from build123d import *

# Parameters (mm, degrees)
F0_W     = 63.6
F0_H     = 31.8
F1_DEPTH = 9.6
F2_W     = 61.2
F2_H     = 29.4
F3_DEPTH = 8.4
F4_R     = 2
F6_DEPTH = 32


with BuildPart() as f1:
    # F0 (on Top) → F1 (new body)
    with BuildSketch(Plane.XY):
        Rectangle(F0_W, F0_H)
    extrude(amount=F1_DEPTH)

    # F2 (on Top) → F3 (cut)
    with BuildSketch(Plane.XY):
        Rectangle(F2_W, F2_H)
    extrude(amount=F3_DEPTH, mode=Mode.SUBTRACT)

    # F4
    f4_edges = [f1.edges().sort_by_distance(p)[0] for p in [
        (-31.8, -15.9, 4.8),
        (-31.8, 15.9, 4.8),
        (31.8, 15.9, 4.8),
        (31.8, -15.9, 4.8),
    ]]
    fillet(f4_edges, radius=F4_R)

    # F5 (on Right) → F6 (cut)
    with BuildSketch(Plane.YZ):
        with BuildLine():
            Line((3.71, 1.5), (-3.71, 1.5))
            ThreePointArc((-3.71, 1.5), (-4.346396, 1.236396), (-4.61, 0.6))
            Line((-4.61, 0.6), (-4.61, -0.6))
            ThreePointArc((-4.61, -0.6), (-4.346396, -1.236396), (-3.71, -1.5))
            Line((-3.71, -1.5), (3.71, -1.5))
            ThreePointArc((3.71, -1.5), (4.346396, -1.236396), (4.61, -0.6))
            Line((4.61, -0.6), (4.61, 0.6))
            ThreePointArc((4.61, 0.6), (4.346396, 1.236396), (3.71, 1.5))
        make_face()
    extrude(amount=F6_DEPTH, mode=Mode.SUBTRACT)


solid = f1.part
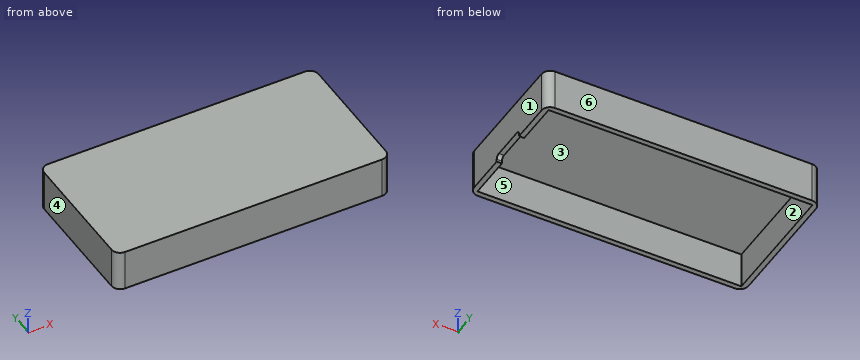
The model under review builds one solid part; all positions refer to its coordinate system, in mm. Face numbers are marked on the shaded views. A direction names the side the tool comes from. Give positions to 0.01 mm unless a question says otherwise; leave off trailing zeros. Order: outer loops, then holes, each group sorted by start corner. A loop starts at its lowest first (then second) coordinate and runs counter-clockwise, first axis right, second up. Notation, with made-up numbers: M 4.5,84 L 23.5,84 A21 ccw 23.5,88 Z; hole C -5.75,13.25 d4. An arc over 180 degrees is marked long. Answer in a Markdown table with one row per item. Add a question column.
1. Machinability: for the marked faces 1 and 2, which of the approach directions +Z, -Z, +X, -X, +Y, -Y give a long, thin tool a straight path to every point of the face, cutting with its end or side? Answer none if there is none.
2. For pin 1 Ø1 at (x, y) = (31, 1) entering from -Z; pin 2 Ø0.7 at (x, z) = (31, 0) entering from -Y; pin 3 Ø8 at (x, y) = (-9, 9.5) entering from -Z, all flat-tipped, find the tip position at first contact; note any pin that passes through.
3. Add section A-A on x = 8. State the section outline as (y, z) points, plus the area to 3 significant figures.
4. Mouldability with a two-part tool opening along X and no side actions: class the marked faces 3, 4, 5 and 6 as released by +X, released by -X, zero draft, split by the parting line, or undercut.
5. To check wall thickness, follow line 1 along X through (y, z) = (12.5, 2.5); line 2 along Y through (x, z) = (2, 4.5); line 3 along Z through (x, y) = (4, 11.5). State the ranges of each line that lie inside material, in increasing order.
6. Add section B-B on y = 8. State the section outline as (x, z) points, plus the area to 3 significant figures.
The answers:
| question | item | result |
|---|---|---|
| 1 | face 1 | +Z, -Z, +X, +Y, -Y |
| 1 | face 2 | -Z |
| 2 | pin 1 | z = 1.5 |
| 2 | pin 2 | y = -15.71 |
| 2 | pin 3 | z = 8.4 |
| 3 | outline | M -15.9,0 L -14.7,0 L -14.7,8.4 L 14.7,8.4 L 14.7,0 L 15.9,0 L 15.9,9.6 L -15.9,9.6 Z |
| 3 | area | 58.3 mm2 |
| 4 | face 3 | undercut |
| 4 | face 4 | released by -X |
| 4 | face 5 | undercut |
| 4 | face 6 | zero draft |
| 5 | line 1 | -31.8 to -30.6, 30.6 to 31.8 |
| 5 | line 2 | -15.9 to -14.7, 14.7 to 15.9 |
| 5 | line 3 | 8.4 to 9.6 |
| 6 | outline | M -31.8,0 L -30.6,0 L -30.6,8.4 L 30.6,8.4 L 30.6,0 L 31.8,0 L 31.8,9.6 L -31.8,9.6 Z |
| 6 | area | 96.5 mm2 |
